Could you check a few things on this drawing? It's one solid part, dimensions in mm from its lowest x, y, z. A direction names the side the tool comes from. Give positions to 0.01 mm unless a question says otherwise; leave off trailing zeros. Loops run counter-clockwise (first coordinate to the right, second up) from the corner with the lowest first, then second, coordinate; pieces in that order, holes last.
1. Imagine slicing it at C-C (x = 12). List the corners of the cut face in (y, z) for me, plus the area to 3 significant figures.
2. Thinking about a two-plate mould opening in Y: for the marked faces 1, 2, 3 and 4, which applies, +Y half, -Y half, draft (parallel to the pull), parting line (faces both ways), or undercut?
3. Imagine slicing it at B-B (y = 48). List the corners of the cut face in (x, z) for me.
4. I need wall thicknesses on line 1 along X through (y, z) = (21, 40); line 2 along Z through (x, y) = (14.5, 35); line 3 along Y through (x, z) = (26, 7.5). Which ranges of each line are inside material? Lowest first, please.
5. Imagine slicing it at D-D (z = 18.5). List the corners of the cut face in (x, y) for me.
6. For P1, Ø25, axis at y = 28.5, z = 57.5, coming from the -X side; P2, Ø1.5, axis at x = 67, y = 32, coming from the -Z side; P3, Ø15, axis at y = 25.5, z = 46.5, coming from the +X side; P4, Ø3, axis at y = 23, z = 3, coming from the -X side, each with a flat end and sliding along its axis, tell me the tip position at first contact or that it passes through.
7. For the marked faces 5, 6 and 7, which set-ups out of +Z, -Z, +X, -X, +Y, -Y let a thin tool reach every point of the face, with its end or its side?
8. Imagine slicing it at A-A (z = 66.5). List the corners of the cut face in (x, y) for me.
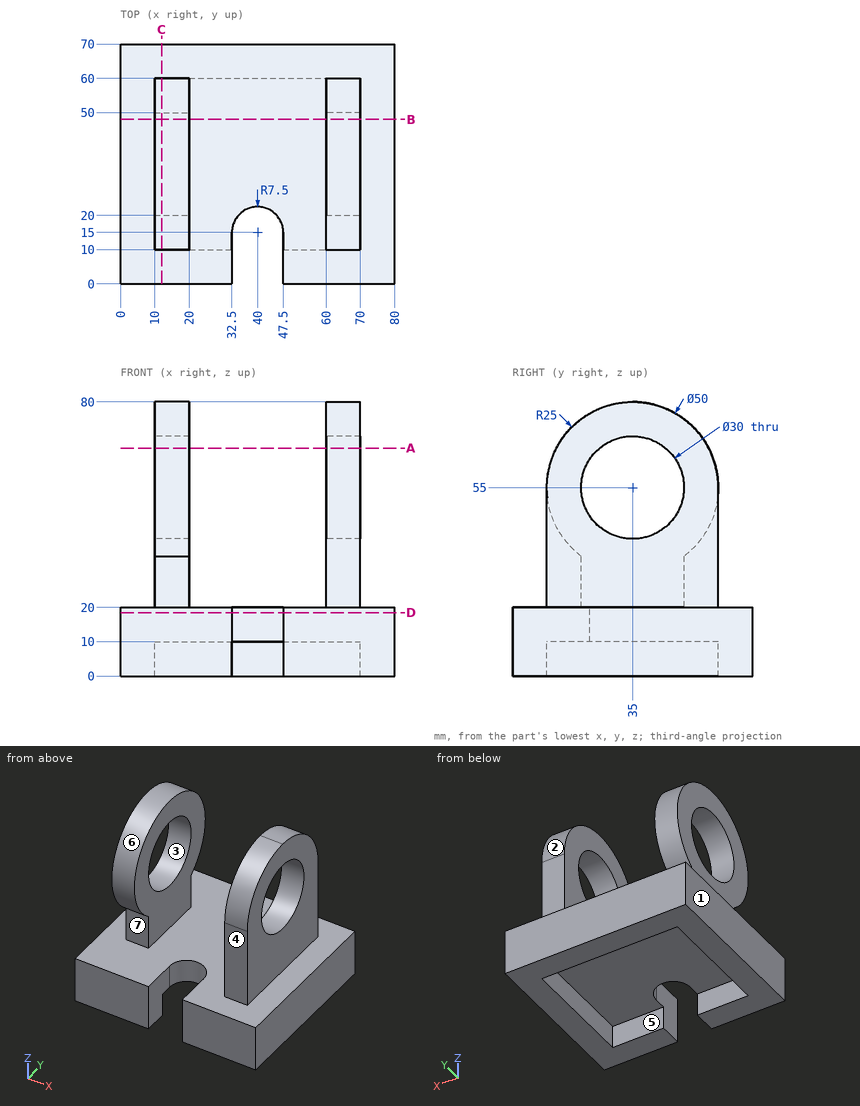
Derived:
1. outline: (0, 0) - (10, 0) - (10, 10) - (60, 10) - (60, 0) - (70, 0) - (70, 20) - (50, 20) - (50, 35) arc R25 ccw (long way) to (20, 35) - (20, 20) - (0, 20) - close; hole circle Ø30 at (35, 55)
1. area: 2,500 mm2
2. face 1: draft
2. face 2: +Y half
2. face 3: undercut
2. face 4: -Y half
3. outline: (0, 0) - (10, 0) - (10, 10) - (70, 10) - (70, 0) - (80, 0) - (80, 20) - (70, 20) - (70, 47.52) - (60, 47.52) - (60, 20) - (20, 20) - (20, 47.52) - (10, 47.52) - (10, 20) - (0, 20) - close; (10, 62.48) - (20, 62.48) - (20, 76.35) - (10, 76.35) - close; (60, 62.48) - (70, 62.48) - (70, 76.35) - (60, 76.35) - close
4. line 1: x = 10 to 20, 60 to 70
4. line 2: z = 10 to 40, 70 to 80
4. line 3: y = 0 to 10, 60 to 70
5. outline: (0, 0) - (32.5, 0) - (32.5, 15) arc R7.5 cw to (47.5, 15) - (47.5, 0) - (80, 0) - (80, 70) - (0, 70) - close
6. P1: stops at x = 10
6. P2: stops at z = 10
6. P3: stops at x = 70
6. P4: stops at x = 0
7. face 5: -Z
7. face 6: -X
7. face 7: -X, -Y
8. outline: (10, 12.8) - (20, 12.8) - (20, 25.37) - (10, 25.37) - close; (10, 44.63) - (20, 44.63) - (20, 57.2) - (10, 57.2) - close; (60, 12.8) - (70, 12.8) - (70, 25.37) - (60, 25.37) - close; (60, 44.63) - (70, 44.63) - (70, 57.2) - (60, 57.2) - close
